Design review of the part built by this model. Coordinates are the model's own, in mm. A direction names the side the tool comes from. Coordinates: 2 decimals unless noted, no trailing zeros. Write each loop counter-clockwise with the first axis right and the second up, starting at its lowest first coordinate (ties: lowest second). Pieces come first, ordered by that corner, then holes.
Q1. Clearance check with flat-ended pins moving along their axes: pin 1 Ø5 at (y, z) = (80, 79) entering from -X; pin 2 Ø2 at (x, z) = (-125, 30.5) entering from +Y; pin 3 Ø4.5 at (y, z) = (80, 109) entering from +X. State where each tip first meets the part, or that it passes through.
Q2. To check wall thickness, follow probe 1 along Y at (x, z) = (-2, 79); probe 2 along Z at (x, y) = (-30, 18); probe 3 along Y at (x, z) = (-134, 48.5). State the ranges of each line that lie inside material, in increasing order.
Q3. The part is to be moulded in two halves that separate along Z. For faces 3 (the face through (-97, 53, 184)), 4 (the face through (-95, 51, 188)), 5 (the face through (-128, 0, 93)), say which applies: +Z half, -Z half, draft (parallel to the pull), parting line (faces both ways), or undercut.
Q4. Add section A-A, the plane y = 40.5. Give the boundary of the cut face in (x, z), plus the area to 3 significant figures.
Q5. Machinability: for faces 1 (the face through (0, 56, 93)), 2 (the face through (-4, 56, 93)), which of the approach directions +Z, -Z, +X, -X, +Y, -Y give a long, thin tool a straight path to every point of the face, cutting with its end or side? Answer none if there is none.
Q6. Add section B-B, the plane z = 40. Give the boundary of the cut face in (x, y), plus the area to 3 significant figures.
from build123d import *

# Parameters (mm, degrees)
DODANIE_WYCI_GNI_CIE1_DEPTH = 188
SKORUPA1_T                  = -4
SZKIC2_R                    = 2
WYTNIJ_WYCI_GNI_CIE1_DEPTH  = 120


with BuildPart() as part:
    # Szkic1 → Dodanie-wyciągnięcie1 (new body)
    with BuildSketch(Plane.XY):
        with BuildLine():
            Line((-10, 0), (-250, 0))
            Line((-250, 0), (-180, 100))
            Line((-180, 100), (0, 100))
            Line((0, 100), (0, 10))
            ThreePointArc((0, 10), (-2.928932188, 2.928932188), (-10, 0))
        make_face()
    extrude(amount=DODANIE_WYCI_GNI_CIE1_DEPTH)

    # Skorupa1
    skorupa1_openings = [part.faces().sort_by_distance(p)[0] for p in [
        (-90, 100, 94),
        (-215, 50, 94),
    ]]
    offset(amount=SKORUPA1_T, openings=skorupa1_openings, kind=Kind.INTERSECTION)

    # Szkic2 → Wytnij-wyciągnięcie1 (cut)
    with BuildSketch(Plane(origin=(0, 0, 0), x_dir=(0, 0, -1), z_dir=(1, 0, 0))):
        with Locations((-109, 80)):
            Circle(SZKIC2_R)
        with Locations((-79, 80)):
            Circle(SZKIC2_R)
        with Locations((-79, 60)):
            Circle(SZKIC2_R)
        with Locations((-109, 60)):
            Circle(SZKIC2_R)
    extrude(amount=-WYTNIJ_WYCI_GNI_CIE1_DEPTH, mode=Mode.SUBTRACT)


solid = part.part
Here are the results:
1. pin 1: stops at x = -4
1. pin 2: stops at y = 4
1. pin 3: stops at x = 0
2. probe 1: y = 4 to 58, 62 to 78, 82 to 100
2. probe 2: z = 0 to 4, 184 to 188
2. probe 3: y = 0 to 4
3. face 3: undercut
3. face 4: +Z half
3. face 5: draft
4. outline: (-221.65, 0) - (0, 0) - (0, 188) - (-221.65, 188) - (-221.65, 184) - (-4, 184) - (-4, 4) - (-221.65, 4) - close
4. area: 2,490 mm2
5. face 1: +Z, -Z, +X, +Y, -Y
5. face 2: -X, +Y
6. outline: (-250, 0) - (-10, 0) arc R10 ccw to (0, 10) - (0, 100) - (-4, 100) - (-4, 10) arc R6 cw to (-10, 4) - (-247.2, 4) - close
6. area: 1,360 mm2
